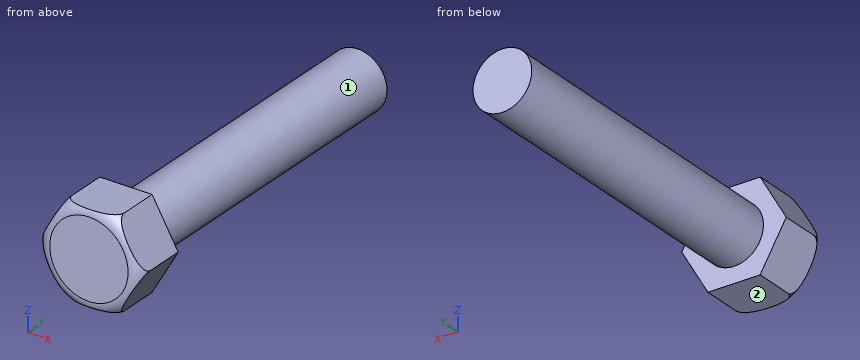
```python
from build123d import *

# Parameters (mm, degrees)
BOSS_EXTRUDE1_DEPTH = 2
SKETCH2_R           = 2.25
BOSS_EXTRUDE2_DEPTH = 25


with BuildPart() as part:
    # Sketch1 → Boss-Extrude1 (new body, symmetric)
    with BuildSketch(Plane(origin=(0, 0, 0), x_dir=(1, 0, 0), z_dir=(0, 1, 0))):
        Polygon((4, 0), (2, 3.464101615), (-2, 3.464101615), (-4, 0), (-2, -3.464101615), (2, -3.464101615), align=None)
    extrude(amount=BOSS_EXTRUDE1_DEPTH, both=True)

    # Sketch2 → Boss-Extrude2 (add)
    with BuildSketch(Plane(origin=(0, 2, 0), x_dir=(1, 0, 0), z_dir=(0, 1, 0))):
        Circle(SKETCH2_R)
    extrude(amount=BOSS_EXTRUDE2_DEPTH)

    # Sketch3 → Cut-Revolve1 (revolve, cut)
    with BuildSketch(Plane.XY):
        with BuildLine():
            Line((2.248897347, -2), (3, -2))
            ThreePointArc((3, -2), (3.707106781, -1.707106781), (4, -1))
            Line((4, -1), (4, -0.81272303))
            Line((4, -0.81272303), (5.594351863, -2.268615273))
            Line((5.594351863, -2.268615273), (3.350773239, -3.273136669))
            Line((3.350773239, -3.273136669), (2.248897347, -2))
        make_face()
    revolve(axis=Axis((0, -2, 0), (0, -1, 0)), mode=Mode.SUBTRACT)


solid = part.part
```
Can you work these out from the model? Positions are in its coordinate system, mm. Face numbers are marked on the shaded views. A direction names the side the tool comes from. Coordinates: 2 decimals unless noted, no trailing zeros. Loops run counter-clockwise (first coordinate to the right, second up) from the corner with the lowest first, then second, coordinate; pieces in that order, holes last. Notation, with made-up numbers: (83, 49) -> (108, 49) arc R15 ccw to (108, 67) -> close; hole circle Ø8 at (-11.5, 6). An arc over 180 degrees is marked (long way). Put each result on its own line as item: value. Start each with the question number.
Q1. I want a section at A-A (x = 0). Write out the boundary of the cut face in (y, z), plus the area to 3 significant figures.
Q2. For the marked faces 1 and 2, which set-ups out of +Z, -Z, +X, -X, +Y, -Y let a thin tool reach every point of the face, with its end or its side?
Q3. I'm going to push flat-ended pins straight in: P1, Ø3, axis at x = -1.5, y = 10, coming from the +Z side; P2, Ø1.5, axis at y = 1.5, z = -2, coming from the +X side; P3, Ø1.5, axis at y = 1.5, z = -2.5, coming from the -X side. Where does each tip first touch, or does it pass through?
Q4. If I drill on line 1 (Y direction, x = -1.25, z = 2.5); line 2 (Y direction, x = -3.5, z = -0.25); line 3 (Z direction, x = 1, y = 9), over which ranges is the centre line in solid material (lowest first)? Write a range as [from, to].
Q5. I want a section at B-B (y = 24.25). Write out the boundary of the cut face in (x, z), plus the area to 3 significant figures.
Taken from the geometry:
1. outline: (-2, -3) arc R1 ccw to (-1.89, -3.46) -> (2, -3.46) -> (2, -2.25) -> (27, -2.25) -> (27, 2.25) -> (2, 2.25) -> (2, 3.46) -> (-1.89, 3.46) arc R1 ccw to (-2, 3) -> close
1. area: 140 mm2
2. face 1: +Y
2. face 2: -Z, +X, -X, +Y, -Y
3. P1: stops at z = 2.25
3. P2: stops at x = 3.28
3. P3: stops at x = -2.99
4. line 1: y = [-2, 2]
4. line 2: y = [-1.86, 2]
4. line 3: z = [-2.02, 2.02]
5. outline: circle Ø4.5 at (0, 0)
5. area: 15.9 mm2
